Part model, mm, in its own coordinate system. A direction names the side the tool comes from. Round coordinates to 2 decimals unless told otherwise and drop trailing zeros. Loops run counter-clockwise (first coordinate to the right, second up) from the corner with the lowest first, then second, coordinate; pieces in that order, holes last. Notation, with made-up numbers: M -7,31.5 L 34,31.5 A27 ccw 34,60.5 Z; hole C 26.5,81 d8. An arc over 180 degrees is marked long. Put each result on its own line as item: value. Start each with the question number.
1) Which spindle directions (+Z, -Z, +X, -X, +Y, -Y) get a long thin tool onto all of the face, cutting with end or side? Do faces 4 (the flat face through (-2.074, -7.741, 4.93)), 5 (the flat face through (-2, 10, 5)), 6 (the flat face through (3, 11, 5)), 7 (the flat face through (-1.4, 7.1, 0)). Say none if no direction does.
2) Slice it at B-B on x = 0. Give the cut face in (y, z), then the cut area to 3 significant figures.
3) Probe line 1 along X through (y, z) = (0, 4.25); line 2 along Y through (x, z) = (0.25, 9.25); line 3 along X through (y, z) = (-3.75, 6.5). List the from-to ranges inside material, lowest first.
4) Slice it at C-C on z = 6.25. Give the cut face in (x, y), then the cut area to 3 significant figures.
5) Pull direction Y, two halves, no side cores. Call faces 1 (the cylindrical face through (8.933, -1.094, 4.93)), 2 (the cylindrical face through (0, 7, 5)), 3 (the flat face through (-3, 11, 5)): +Y half, -Y half, draft (parallel to the pull), parting line (faces both ways), or undercut.
6) Drop flat-ended pins along their axis: pin 1 Ø4.5 at (y, z) = (11.5, 3) entering from +X; pin 2 Ø2.5 at (y, z) = (11, 7) entering from +X; pin 3 Ø3 at (x, z) = (-5, 7.5) entering from +Y; pin 4 Ø2 at (x, y) = (-3.5, 3.5) entering from +Z. Give the stop position or say it passes through.
7) Slice it at A-A on y = 0. Give the cut face in (x, z), then the cut area to 3 significant figures.
```python
from build123d import *

# Parameters (mm, degrees)
PAD_DEPTH    = 10
SKETCH001_W  = 6
SKETCH001_H  = 5.514719
PAD001_DEPTH = 10
FILLET_R     = 2
SKETCH002_W  = 4
SKETCH002_H  = 4
POCKET_DEPTH = 10.001


with BuildPart() as part:
    # Sketch → Pad (new body)
    with BuildSketch(Plane.XY):
        with BuildLine():
            ThreePointArc((2.329371, -8.693332), (0, 9), (-2.329371, -8.693332))
            Line((-2.329371, -8.693332), (-1.811733, -6.761481))
            ThreePointArc((1.811733, -6.761481), (0, 7), (-1.811733, -6.761481))
            Line((1.811733, -6.761481), (2.329371, -8.693332))
        make_face()
    extrude(amount=PAD_DEPTH)

    # Sketch001 (on Face6 of Pad) → Pad001 (join)
    with BuildSketch(Plane.XY.offset(10)):
        with Locations((0, 11.242641)):
            Rectangle(SKETCH001_W, SKETCH001_H)
    extrude(amount=-PAD001_DEPTH)

    # Fillet
    fillet_edges = [part.edges().sort_by_distance(p)[0] for p in [
        (-3, 14, 5),
        (0, 14, 0),
        (3, 14, 5),
        (3, 8.485281, 5),
        (-3, 8.485281, 5),
    ]]
    fillet(fillet_edges, radius=FILLET_R)

    # Sketch002 (on Face18 of Fillet) → Pocket (cut, through all)
    with BuildSketch(Plane.XY.offset(10)):
        with Locations((0, 10.5)):
            Rectangle(SKETCH002_W, SKETCH002_H)
    extrude(amount=-POCKET_DEPTH, mode=Mode.SUBTRACT)


solid = part.part
```
Recorded:
1. face 4: +Z, -Z, -Y
1. face 5: +Z, -Z
1. face 6: +Z, -Z, +X, +Y
1. face 7: -Z, +X, -X, +Y, -Y
2. outline: M 7,0 L 8.5,0 L 8.5,10 L 7,10 Z; M 12.5,0.06 A2 ccw 14,2 L 14,10 L 12.5,10 Z
2. area: 29.2 mm2
3. line 1: x = -9 to -7, 7 to 9
3. line 2: y = 7 to 8.5, 12.5 to 14
3. line 3: x = -8.18 to -5.91, 5.91 to 8.18
4. outline: M -4.09,8.02 A9 ccw -2.33,-8.69 L -1.81,-6.76 A7 cw long 1.81,-6.76 L 2.33,-8.69 A9 ccw 4.09,8.02 A2 cw 3,9.8 L 3,12 A2 ccw 1,14 L -1,14 A2 ccw -3,12 L -3,9.8 A2 cw Z; hole M -2,8.5 L 2,8.5 L 2,12.5 L -2,12.5 Z
4. area: 106 mm2
5. face 1: parting line
5. face 2: undercut
5. face 3: draft
6. pin 1: stops at x = 3.08
6. pin 2: stops at x = 3
6. pin 3: stops at y = 8.48
6. pin 4: passes through
7. outline: M -9,0 L -7,0 L -7,10 L -9,10 Z; M 7,0 L 9,0 L 9,10 L 7,10 Z
7. area: 40.0 mm2
